The listing builds one solid part. Answer for the finished solid, in the listing's coordinates (mm). Face numbers are marked on the shaded views. A direction names the side the tool comes from. Coordinates: 2 decimals unless noted, no trailing zeros. Order: outer loops, then holes, each group sorted by start corner. A loop starts at its lowest first (then second) coordinate and runs counter-clockwise, first axis right, second up. Notation, with made-up numbers: (-9.75, 65.5) -> (9.25, 65.5) arc R14 cw to (9.25, 69.5) -> close; hole circle Ø3 at (2.5, -36.5). An arc over 180 degrees is marked (long way). Write each question's results on one line, items separated by ' | '. Start each with the question number.
(1) A tool of negligible diameter and unlimited length cuts with its end or side. For the marked faces 1, 2 and 3, from which of +Z, -Z, +X, -X, +Y, -Y can it reach the whole face along a straight path? Write none if from no direction.
(2) The part is cut by section A-A, the plane x = -28. Give the vertices of the cut face in (y, z).
(3) The part is cut by section C-C, the plane y = 143. Give the vertices of the cut face in (x, z) (3 decimals).
(4) The part is cut by section B-B, the plane z = 90. Give the vertices of the cut face in (x, y) (3 decimals), then the cut area to 3 significant figures.
(5) Given pin 1 (3 mm diameter, centred on x = 71.5, z = 63, fed in from +Y); pin 2 (10 mm diameter, centred on x = -13.5, y = 65, fed in from +Z); pin 3 (14 mm diameter, centred on x = -48.5, z = 93.5, fed in from +Y), each flat-ended and moving along its own axis, determine where each tip first touches the part or whether it passes through.
(6) Determine the mould class of the marked faces 4, 5, 6 and 7 for opening direction Z: +Z half, -Z half, draft (parallel to the pull), parting line (faces both ways), or undercut.
(7) The part is cut by section D-D, the plane x = 11. Give the vertices of the cut face in (y, z), then the cut area to 3 significant figures.
(8) Straight lines are drawn through the part: L1, parallel to Z at x = 77.5, y = 84.5; L2, parallel to Z at x = 63.5, y = 71.5; L3, parallel to Y at x = 59.5, z = 120. For each, find the intervals that lie inside material, in ascending order.
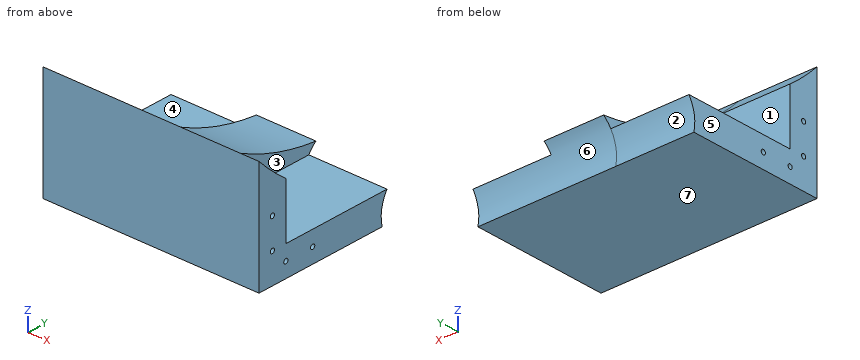
Autodesk Inventor part; units mm, degrees
ref_plane "YZ Plane" through (0, 0, 0) normal (1, 0, 0) x (0, 1, 0)
ref_plane "XZ Plane" through (0, 0, 0) normal (0, 1, 0) x (-1, 0, 0)
ref_plane "XY Plane" through (0, 0, 0) normal (0, 0, 1) x (1, 0, 0)
sketch "Sketch1" plane through (0, 0, 0) normal (1, 0, 0) x (0, 1, 0)
  circle A0 centre (180.7797, 284.5338) radius 25.4
  line L0 (-17.3403, 309.9338) -> (-51.2615, 309.9338)
  line L1 (-51.2615, 309.9338) -> (-51.2615, -502.8662)
  line L2 (-51.2615, -502.8662) -> (-17.3403, -502.8662)
  line L3 (-17.3403, -502.8662) -> (-17.3403, 309.9338)
  line L4 (33.4597, 146.4304) -> (33.4597, 50.9549)
  arc A1 (202.8525, 71.0418) -> (198.1508, 77.005) centre (180.7797, 58.4738) ccw
  line L5 (198.1508, 7.6738) -> (231.5797, 7.6738)
  line L6 (231.5797, 7.6738) -> (231.5797, 309.9338)
  line L7 (231.5797, 309.9338) -> (33.4597, 309.9338)
  line L8 (33.4597, 146.4304) -> (33.4597, 50.9549)
  line L9 (198.1508, 76.3549) -> (198.1508, 50.9549)
  line L10 (33.4597, 50.9549) -> (33.4597, 76.3549)
  line L11 (33.4597, 50.9549) -> (58.8597, 50.9549)
  line L12 (33.4597, 119.3221) -> (33.4597, 50.9549)
  line L13 (149.9329, 50.9549) -> (33.4597, 50.9549)
  arc A2 (231.5797, 89.0982) -> (-17.3403, 245.4929) centre (180.7797, 284.5338) ccw
  arc A3 (33.4597, 146.4304) -> (161.2998, 83.5456) centre (180.7797, 284.5338) ccw
  arc A4 (161.2998, 83.5456) -> (149.9329, 50.9549) centre (180.7797, 58.4738) ccw
  arc A5 (198.1508, 70.6079) -> (202.8525, 71.0418) centre (180.7797, 284.5338) ccw
  arc A6 (231.5797, 76.0023) -> (-17.3403, 201.9838) centre (180.7797, 284.5338) ccw
  point P0 (0, 0)
  dimension "d1" = 50.8
  dimension "d2" = 812.8
  dimension "d5" = 25.4
  dimension "d6" = 198.12
  dimension "d10" = 50.8
  dimension "d11" = 50.8
  dimension "d12" = 226.06
  dimension "d15" = 25.4
  dimension "d16" = 50.8
  dimension "d17" = 302.26
  dimension "d18" = 50.8
extrude "Extrusion1" add sketch "Sketch1" along normal blind 50.8 contours A3 A4 L13 L11 L4
sketch "Sketch2" plane through (50.8, 0, 0) normal (1, 0, 0) x (0, 0, -1)
  line L0 (-146.4304, 33.4597) -> (-50.9549, 33.4597)
  line L1 (-50.9549, 33.4597) -> (-146.4304, 33.4597)
  line L2 (-123.5641, 58.8597) -> (-76.3549, 58.8597)
  line L3 (-50.9549, 58.8597) -> (-50.9549, 33.4597)
  line L4 (-50.9549, 33.4597) -> (-76.3549, 33.4597)
  line L5 (-76.3549, 58.8597) -> (-76.3549, 154.5437)
  line L6 (-50.9549, 149.9329) -> (-50.9549, 33.4597)
  arc A0 (-146.4304, 33.4597) -> (-83.5456, 161.2998) centre (-284.5338, 180.7797) ccw
  arc A1 (-83.5456, 161.2998) -> (-50.9549, 149.9329) centre (-58.4738, 180.7797) ccw
  line L7 (-50.9549, 33.4597) -> (-50.9549, 149.9329)
  arc A2 (-76.3549, 154.5437) -> (-50.9549, 149.9329) centre (-58.4738, 180.7797) ccw
  arc A3 (-146.4304, 33.4597) -> (-123.5641, 58.8597) centre (-284.5338, 180.7797) ccw
  point P0 (0, 0)
  dimension "d30" = 25.4
  dimension "d31" = 25.4
extrude "Extrusion2" add sketch "Sketch2" along normal blind 66.675 contours A0 L2 L5 A1 L6 L3 L0
sketch "Sketch3" plane through (0, 0, 0) normal (-1, 0, 0) x (0, 0, 1)
  line L0 (76.3549, 58.8597) -> (76.3549, 154.5437)
  arc A0 (50.9549, 149.9329) -> (83.5456, 161.2998) centre (58.4738, 180.7797) ccw
  line L1 (50.9549, 33.4597) -> (50.9549, 149.9329)
  line L2 (146.4304, 33.4597) -> (50.9549, 33.4597)
  arc A1 (83.5456, 161.2998) -> (146.4304, 33.4597) centre (284.5338, 180.7797) ccw
  line L3 (123.5641, 58.8597) -> (76.3549, 58.8597)
  line L4 (76.3549, 154.5437) -> (76.3549, 58.8597)
  line L5 (76.3549, 154.5437) -> (76.3549, 58.8597)
  line L6 (76.3549, 58.8597) -> (123.5641, 58.8597)
  line L7 (50.9549, 149.9329) -> (50.9549, 33.4597)
  line L8 (146.4304, 33.4597) -> (50.9549, 33.4597)
  arc A2 (50.9549, 149.9329) -> (76.3549, 154.5437) centre (58.4738, 180.7797) ccw
  arc A3 (123.5641, 58.8597) -> (146.4304, 33.4597) centre (284.5338, 180.7797) ccw
  point P0 (0, 0)
extrude "Extrusion3" add sketch "Sketch3" along normal blind 66.675 contours L3 A1 L2 L1 A0 L0
sketch "Sketch4" plane through (117.475, 0, 0) normal (1, 0, 0) x (0, 0, -1)
  line L0 (-146.4304, 33.4597) -> (-50.9549, 33.4597)
  line L1 (-50.9549, 33.4597) -> (-50.9549, 149.9329)
  point P0 (0, 0)
  point P1 (-76.3549, 46.1597)
  point P2 (-101.7549, 46.1597)
  point P3 (-63.6549, 58.8597)
  point P4 (-63.6549, 84.2597)
  dimension "d36" = 0
  dimension "d37" = 25.4
  dimension "d38" = 25.4
  dimension "d39" = 0
  dimension "d40" = 25.4
  dimension "d41" = 25.4
  dimension "d42" = 12.7
  dimension "d43" = 12.7
hole "Hole1" at (117.475, 46.1597, 76.3549) at (117.475, 46.1597, 101.7549) at (117.475, 58.8597, 63.6549) at (117.475, 84.2597, 63.6549) direction (-1, 0, 0) diameter 3.9624 end through all
properties part number "BottomRamp"
Established:
1) face 1: +Z, -X, +Y | face 2: +X, -X, +Y | face 3: +Z, +X, +Y
2) outline: (33.46, 50.95) -> (149.93, 50.95) arc R31.75 cw to (154.54, 76.35) -> (58.86, 76.35) -> (58.86, 123.56) arc R201.93 cw to (33.46, 146.43) -> close; hole circle Ø3.96 at (46.16, 76.35); hole circle Ø3.96 at (46.16, 101.75); hole circle Ø3.96 at (58.86, 63.65); hole circle Ø3.96 at (84.26, 63.65)
3) outline: (-66.675, 50.955) -> (117.475, 50.955) -> (117.475, 76.355) -> (50.8, 76.355) -> (50.8, 86.169) -> (0, 86.169) -> (0, 76.355) -> (-66.675, 76.355) -> close
4) outline: (-66.675, 33.46) -> (117.475, 33.46) -> (117.475, 58.86) -> (50.8, 58.86) -> (50.8, 126.629) -> (0, 126.629) -> (0, 58.86) -> (-66.675, 58.86) -> close | area: 8,120 mm^2
5) pin 1: stops at y = 149.61 | pin 2: stops at z = 76.35 | pin 3: stops at y = 58.86
6) face 4: +Z half | face 5: draft | face 6: undercut | face 7: -Z half
7) outline: (33.46, 50.95) -> (149.93, 50.95) arc R31.75 cw to (161.3, 83.55) arc R201.93 cw to (33.46, 146.43) -> close; hole circle Ø3.96 at (46.16, 76.35); hole circle Ø3.96 at (46.16, 101.75); hole circle Ø3.96 at (58.86, 63.65); hole circle Ø3.96 at (84.26, 63.65) | area: 6,590 mm^2
8) L1: z = 50.95 to 61.69, 65.62 to 76.35 | L2: z = 50.95 to 76.35 | L3: y = 33.46 to 58.86
